Geometry check sheet. Reference: the model listing, model coordinates, mm. Round coordinates to 2 decimals unless told otherwise and drop trailing zeros. Loops run counter-clockwise (first coordinate to the right, second up) from the corner with the lowest first, then second, coordinate; pieces in that order, holes last. Notation, with made-up numbers: (-8, -10) -> (15, -10) arc R26 ccw to (15, 28) -> close; hole circle Ø3 at (7.25, 4.5). An arc over 180 degrees is marked (long way). Use one line per item in the form item = value.
Autodesk Inventor part; units mm, degrees
ref_plane "YZ Plane" through (0, 0, 0) normal (1, 0, 0) x (0, 1, 0)
ref_plane "XZ Plane" through (0, 0, 0) normal (0, 1, 0) x (-1, 0, 0)
ref_plane "XY Plane" through (0, 0, 0) normal (0, 0, 1) x (1, 0, 0)
sketch "Sketch2" plane through (0, 0, 0) normal (0, 0, 1) x (1, 0, 0)
  line L0 (-75, -25) -> (75, -25)
  line L1 (75, -25) -> (75, 25)
  line L2 (75, 25) -> (-75, 25)
  line L3 (-75, 25) -> (-75, -25)
  line L4 (-75, -25) -> (75, 25) construction
  line L5 (75, -25) -> (-75, 25) construction
  point P0 (0, 0)
  dimension "d1" = 150
  dimension "d2" = 50
extrude "Extrusion1" add sketch "Sketch2" along normal mid plane 10
sketch "Sketch3" plane through (0, 0, 5) normal (0, 0, 1) x (1, 0, 0)
  line L0 (-75, 25) -> (-75, -25)
  line L1 (75, 25) -> (-75, 25)
  point P0 (0, 0)
  point P1 (-65, 0)
  dimension "d40" = 10
  dimension "d43" = 25
hole "Hole1" at (-65, 0, 5) direction (0, 0, -1) diameter 5.5 depth 14.2 tip angle 118
sketch "Sketch4" plane through (0, 0, 5) normal (0, 0, 1) x (1, 0, 0)
  line L0 (-75, 25) -> (-75, -25)
  line L1 (75, 25) -> (-75, 25)
  point P0 (0, 0)
  point P1 (-45, 5)
  dimension "d41" = 30
  dimension "d42" = 20
hole "Hole2" at (-45, 5, 5) direction (0, 0, -1) diameter 6.6 depth 14.2 tip angle 118
sketch "Sketch5" plane through (0, 0, 5) normal (0, 0, 1) x (1, 0, 0)
  line L0 (-75, 25) -> (-75, -25)
  line L1 (75, 25) -> (-75, 25)
  point P0 (0, 0)
  point P1 (-24, 5)
  dimension "d44" = 51
  dimension "d45" = 20
hole "Hole3" at (-24, 5, 5) direction (0, 0, -1) diameter 9 depth 14.2 tip angle 118
sketch "Sketch6" plane through (0, 0, 5) normal (0, 0, 1) x (1, 0, 0)
  line L0 (-75, 25) -> (-75, -25)
  line L1 (75, 25) -> (-75, 25)
  point P0 (0, 0)
  point P1 (5, 5)
  dimension "d46" = 80
  dimension "d47" = 20
hole "Hole4" at (5, 5, 5) direction (0, 0, -1) diameter 6 depth 14.2 tip angle 118
sketch "Sketch7" plane through (0, 0, 5) normal (0, 0, 1) x (1, 0, 0)
  line L0 (-75, 25) -> (-75, -25)
  line L1 (75, 25) -> (-75, 25)
  point P0 (0, 0)
  point P1 (25, 5)
  dimension "d48" = 100
  dimension "d49" = 20
hole "Hole5" at (25, 5, 5) direction (0, 0, -1) diameter 10 depth 14.2 tip angle 118
pattern_linear "Rectangular Pattern1" count 3 spacing 11 along (0, -1, 0) of "Hole1" first direction both ways yes
pattern_linear "Rectangular Pattern2" count 2 spacing 10 along (0, -1, 0) of "Hole2"
pattern_linear "Rectangular Pattern3" count 2 spacing 14.5 along (0, -1, 0) of "Hole3"
pattern_linear "Rectangular Pattern4" count 3 spacing 10 along (0, -1, 0) of "Hole4"
pattern_linear "Rectangular Pattern5" count 2 spacing 20 along (0, -1, 0) of "Hole5"
properties part number "홀간 거리 확인 파트-9" material "SS400"
1. Material ranges on line 1 along Y through (x, z) = (-24, -1); line 2 along Y through (x, z) = (5, 2.5); line 3 along X through (y, z) = (5, 1.25), recorded low to high.
Return value:
line_1 = -25 to -14, -5 to 0.5, 9.5 to 25
line_2 = -25 to -18, -12 to -8, -2 to 2, 8 to 25
line_3 = -75 to -48.3, -41.7 to -28.5, -19.5 to 2, 8 to 20, 30 to 75
2. Section check C-C (y = 5). Record the boundary of the cut face in (x, z), then the cut area to 3 significant figures.
Return value:
outline = (-75, -5) -> (-48.3, -5) -> (-48.3, 5) -> (-75, 5) -> close; (-41.7, -5) -> (-28.5, -5) -> (-28.5, 5) -> (-41.7, 5) -> close; (-19.5, -5) -> (2, -5) -> (2, 5) -> (-19.5, 5) -> close; (8, -5) -> (20, -5) -> (20, 5) -> (8, 5) -> close; (30, -5) -> (75, -5) -> (75, 5) -> (30, 5) -> close
area = 1,180 mm2
3. Mould release check, pull along X, two halves, no side actions. Record for faces 1 (the cylindrical face through (2, -5, 0)), 2 (the cylindrical face through (2.97, -12.79, -0.07)), 3 (the flat face through (75, 0, 0)), 4 (the flat face through (-1, 0, 5)): released by +X, released by -X, zero draft, split by the parting line, or undercut.
Return value:
face_1 = undercut
face_2 = undercut
face_3 = released by +X
face_4 = zero draft
4. Section check A-A (z = -3.25). Count the separate pieces of the cut face and the enclosed holes in it, then the cut area to 3 significant figures.
Return value:
separate_pieces = 1
enclosed_holes = 12
area = 6,990 mm2
5. Section check D-D (x = -45). Record the boundary of the cut face in (y, z), then the cut area to 3 significant figures.
Return value:
outline = (-25, -5) -> (-8.3, -5) -> (-8.3, 5) -> (-25, 5) -> close; (-1.7, -5) -> (1.7, -5) -> (1.7, 5) -> (-1.7, 5) -> close; (8.3, -5) -> (25, -5) -> (25, 5) -> (8.3, 5) -> close
area = 368 mm2
6. Gauge pin test, flat end, axial feed: pin 1 (8 mm diameter, centred on x = 25, y = -15, fed in from +Z). Record the tip position at first contact, or that the pin passes through.
Return value:
pin_1 = through
7. Section check B-B (x = -65). Record the boundary of the cut face in (y, z), then the cut area to 3 significant figures.
Return value:
outline = (-25, -5) -> (-13.75, -5) -> (-13.75, 5) -> (-25, 5) -> close; (-8.25, -5) -> (-2.75, -5) -> (-2.75, 5) -> (-8.25, 5) -> close; (2.75, -5) -> (8.25, -5) -> (8.25, 5) -> (2.75, 5) -> close; (13.75, -5) -> (25, -5) -> (25, 5) -> (13.75, 5) -> close
area = 335 mm2
